Autodesk Fusion 360 part; units mm, degrees
sketch "Sketch1" plane through (0, 0, 0) normal (0, 0, 1) x (1, 0, 0)
  line L0 (13.6, 14.175) -> (-13.6, 14.175)
  line L1 (-13.6, 14.175) -> (-13.6, -14.175)
  line L2 (-13.6, -14.175) -> (13.6, -14.175)
  line L3 (13.6, -14.175) -> (13.6, 14.175)
  line L4 (13.6, 14.175) -> (-13.6, -14.175) construction
  line L5 (-13.6, 14.175) -> (13.6, -14.175) construction
  line L6 (-7.075, 14.175) -> (7.075, 14.175)
  line L7 (7.075, 14.175) -> (7.075, 12.175)
  line L8 (7.075, 12.175) -> (-7.075, 12.175)
  line L9 (-7.075, 12.175) -> (-7.075, 14.175)
  line L10 (-13.6, 9.675) -> (13.6, 9.675)
  line L11 (13.6, 9.675) -> (13.6, -9.075)
  line L12 (13.6, -9.075) -> (-13.6, -9.075)
  line L13 (-13.6, -9.075) -> (-13.6, 9.675)
  line L14 (-13.6, 5.675) -> (13.6, 5.675)
  circle A0 centre (12.0919, 12.6032) radius 1.375
  circle A1 centre (-4.5, -12.675) radius 1
  circle A2 centre (-4.5, -12.675) radius 1
  circle A3 centre (-1.5, -12.675) radius 1
  circle A4 centre (1.5, -12.675) radius 1
  circle A5 centre (4.5, -12.675) radius 1
  line L15 (-4.5, -12.675) -> (4.5, -12.675) construction
  line L16 (0, -14.175) -> (0, -11.175) construction
  circle A6 centre (-4.5, -12.675) radius 0.5
  circle A7 centre (-1.5, -12.675) radius 0.5
  circle A8 centre (1.5, -12.675) radius 0.5
  circle A9 centre (4.5, -12.675) radius 0.5
  circle A10 centre (-12.1081, 12.6032) radius 1.375
  circle A11 centre (12.0919, -12.5968) radius 1.375
  circle A12 centre (-12.1081, -12.5968) radius 1.375
  dimension "d1" = 27.2
  dimension "d2" = 28.35
  dimension "d3" = 14.15
  dimension "d4" = 2
  dimension "d5" = 18.75
  dimension "d6" = 4.5
  dimension "d7" = 4
  dimension "d8" = 2.75
  dimension "d22" = 2
  dimension "d23" = 2
  dimension "d26" = 3
  dimension "d27" = 0
  dimension "d30" = 3
  dimension "d31" = 1
  dimension "d36" = -24.2
  dimension "d37" = -25.2
extrude "Extrude1" add sketch "Sketch1" against normal blind 1.15 contours L0 L1 L3 L7 L8 L9 L10 | L1 L3 L10 L11 L13 L14 | L1 L3 L11 L12 L13 L14 | L1 L2 L3 L12 | A1 A2 | A3 | A4 | A5
extrude "Extrude2" add sketch "Sketch1" along normal blind 1.15 contours L1 L3 L10 L11 L13 L14
extrude "Extrude3" add sketch "Sketch1" along normal blind 1.2 contours L1 L3 L11 L12 L13 L14
sketch "Sketch2" plane through (13.6, 0, 0) normal (1, 0, 0) x (0, 1, 0)
  line L0 (-9.075, 0) -> (-14.175, 0)
  line L1 (-14.175, 0) -> (-14.175, -1.15)
  line L2 (-14.175, -1.15) -> (14.175, -1.15)
  line L3 (14.175, -1.15) -> (14.175, 0)
  line L4 (14.175, 0) -> (9.675, 0)
  line L5 (9.675, 0) -> (9.675, 1.15)
  line L6 (9.675, 1.15) -> (5.675, 1.15)
  line L7 (5.675, 1.15) -> (5.675, 1.2)
  line L8 (5.675, 1.2) -> (-9.075, 1.2)
  line L9 (-9.075, 1.2) -> (-9.075, 0)
  line L10 (-9.075, 0) -> (9.675, 0)
extrude "Extrude4" add sketch "Sketch2" along normal blind 0.01 contours L0 L1 L2 L3 L4 L10
sketch "Sketch3" plane through (-13.6, 0, 0) normal (-1, 0, 0) x (0, -1, 0)
  line L0 (-9.675, 0) -> (-14.175, 0)
  line L1 (-14.175, 0) -> (-14.175, -1.15)
  line L2 (-14.175, -1.15) -> (14.175, -1.15)
  line L3 (14.175, -1.15) -> (14.175, 0)
  line L4 (14.175, 0) -> (9.075, 0)
  line L5 (9.075, 0) -> (9.075, 1.2)
  line L6 (9.075, 1.2) -> (-5.675, 1.2)
  line L7 (-5.675, 1.2) -> (-5.675, 1.15)
  line L8 (-5.675, 1.15) -> (-9.675, 1.15)
  line L9 (-9.675, 1.15) -> (-9.675, 0)
  line L10 (-9.675, 0) -> (9.075, 0)
extrude "Extrude5" add sketch "Sketch3" along normal blind 0.01 contours L0 L1 L2 L3 L4 L10
extrude "Extrude6" cut sketch "Sketch1" against normal blind 0.01 contours A1 A2 | A3 | A4 | A5
equation "d26 = 1 mm + 2 mm"
Could you check a few things on this model? Use its own coordinates, in mm. Give positions to 0.01 mm unless a question says otherwise; leave off trailing zeros. Write each loop counter-clockwise with the first axis right and the second up, starting at its lowest first coordinate (ties: lowest second). Pieces come first, ordered by that corner, then holes. Notation, with made-up numbers: (38.25, 67) -> (50.25, 67) arc R32 cw to (50.25, 106) -> close; hole circle Ø4 at (31, 3.5). An arc over 180 degrees is marked (long way). Write each question's results on one line, items separated by ' | '.
1. Will these pins go through, and if not, where does the flat tip stop? pin 1 Ø0.9 at (x, z) = (-6, 0.5) entering from +Y (3 decimals); pin 2 Ø1.6 at (x, y) = (-1.5, -12.675) entering from +Z; pin 3 Ø2 at (x, y) = (1.5, 7) entering from +Z; pin 4 Ø3 at (x, y) = (-4.5, -12.675) entering from -Z.
Check sheet entries:
pin 1: stops at y = 9.675 | pin 2: stops at z = -0.01 | pin 3: stops at z = 1.15 | pin 4: stops at z = -1.15
2. I want a section at A-A, the plane x = 1.5. Write out the boundary of the cut face in (y, z) (3 decimals).
Check sheet entries:
outline: (-14.175, -1.15) -> (-13.175, -1.15) -> (-13.175, -0.01) -> (-13.675, -0.01) -> (-13.675, 0) -> (-14.175, 0) -> close; (-12.175, -1.15) -> (12.175, -1.15) -> (12.175, 0) -> (9.675, 0) -> (9.675, 1.15) -> (5.675, 1.15) -> (5.675, 1.2) -> (-9.075, 1.2) -> (-9.075, 0) -> (-11.675, 0) -> (-11.675, -0.01) -> (-12.175, -0.01) -> close
3. I need wall thicknesses on L1, parallel to Y at x = -1.5, z = -0.9 (3 decimals); L2, parallel to Z at x = 9, y = 9.75; L3, parallel to X at y = -2.75, z = 0.5. Which ranges of each line are inside material? Lowest first, please.
Check sheet entries:
L1: y = -14.175 to -13.175, -12.175 to 12.175 | L2: z = -1.15 to 0 | L3: x = -13.6 to 13.6
4. I want a section at B-B, the plane x = -7.5. Write out the boundary of the cut face in (y, z) (3 decimals), then the cut area to 3 significant figures.
Check sheet entries:
outline: (-14.175, -1.15) -> (14.175, -1.15) -> (14.175, 0) -> (9.675, 0) -> (9.675, 1.15) -> (5.675, 1.15) -> (5.675, 1.2) -> (-9.075, 1.2) -> (-9.075, 0) -> (-14.175, 0) -> close | area: 54.9 mm²
5. If we mould it in two halves opening along Y, with no side actions, what happens to faces 1 (the flat face through (0, 0, -1.15)), 2 (the cylindrical face through (11.078, 13.532, -0.567)), 3 (the flat face through (0.1, 12.175, -0.6))? For each: released by +Y, released by -Y, zero draft, split by the parting line, or undercut.
Check sheet entries:
face 1: zero draft | face 2: undercut | face 3: released by +Y
6. I want a section at D-D, the plane z = -0.75. Count the separate pieces of the cut face and the enclosed holes in it, then the cut area to 3 significant figures.
Check sheet entries:
separate pieces: 1 | enclosed holes: 8 | area: 716 mm²
